Autodesk Inventor part; units mm, degrees
ref_plane "YZ Plane" through (0, 0, 0) normal (1, 0, 0) x (0, 1, 0)
ref_plane "XZ Plane" through (0, 0, 0) normal (0, 1, 0) x (-1, 0, 0)
ref_plane "XY Plane" through (0, 0, 0) normal (0, 0, 1) x (1, 0, 0)
sketch "Sketch1" plane through (0, 0, 0) normal (0, 1, 0) x (-1, 0, 0)
  line L0 (0, 0) -> (-30.48, 0)
  line L1 (-30.48, 0) -> (-30.48, -15.24)
  line L2 (-30.48, -15.24) -> (0, -15.24)
  line L3 (0, -15.24) -> (0, 0)
  line L4 (0, -7.62) -> (-30.48, -7.62) construction
  circle A0 centre (-7.874, -7.62) radius 1.143
  circle A1 centre (-22.606, -7.62) radius 1.143
  dimension "d0" = 15.24
  dimension "d1" = 30.48
  dimension "d2" = 2.286
  dimension "d3" = 2.286
  dimension "d4" = 14.732
  dimension "d5" = 7.874
extrude "Extrusion1" add sketch "Sketch1" along normal blind 2.032
sketch "Sketch2" plane through (0, 2.032, 0) normal (0, 1, 0) x (1, 0, 0)
  line L0 (0, 0) -> (30.48, 0)
  line L1 (30.48, 0) -> (30.48, 15.24)
  line L2 (30.48, 15.24) -> (0, 15.24)
  line L3 (0, 15.24) -> (0, 0)
  line L4 (2.032, 2.032) -> (28.448, 2.032)
  line L5 (28.448, 2.032) -> (28.448, 13.208)
  line L6 (28.448, 13.208) -> (2.032, 13.208)
  line L7 (2.032, 13.208) -> (2.032, 2.032)
  dimension "d8" = 2.032
  dimension "d9" = 2.032
  dimension "d10" = 2.032
  dimension "d12" = 2.032
extrude "Extrusion2" add sketch "Sketch2" along normal blind 0.9398
properties part number "castor_bracket"
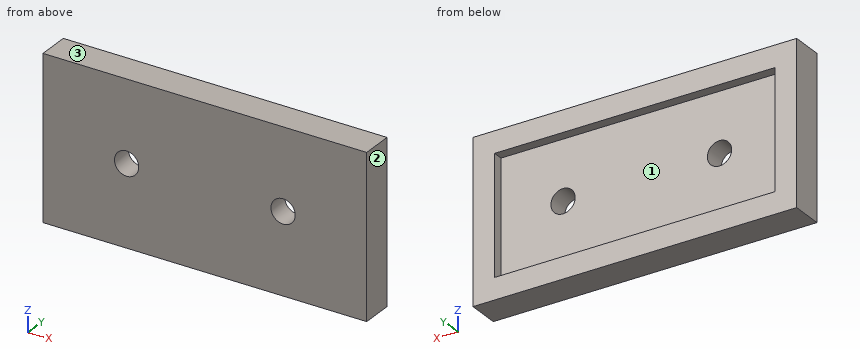
Design review of the part built by this model. Coordinates are the model's own, in mm. Face numbers are marked on the shaded views. Round coordinates to 2 decimals unless told otherwise and drop trailing zeros. Loops run counter-clockwise (first coordinate to the right, second up) from the corner with the lowest first, then second, coordinate; pieces in that order, holes last. Notation, with made-up numbers: (35, 19.5) -> (58, 19.5) arc R23 ccw to (58, 58.5) -> close; hole circle Ø11 at (77.25, -33.5). An arc over 180 degrees is marked (long way). Use one line per item in the form item = value. Start each with the question number.
Q1. We need section A-A on z = -7.62. Give the boundary of the cut face in (x, y).
Q2. We need section B-B on x = 22. Give the boundary of the cut face in (y, z).
Q3. We need section D-D on y = 2.35. Give the boundary of the cut face in (x, z).
Q4. Wall thickness on line 1 along Z through (x, y) = (23.5, 2.8); line 2 along Y through (x, z) = (11.5, -12.25): over which ranges is each line inside the solid? List them lowest first. Write a range as [from, to].
Q5. For pin 1 Ø3 at (x, z) = (6, -10) entering from +Y; pin 2 Ø8 at (x, z) = (25.5, -8) entering from -Y; pin 3 Ø1.4 at (x, z) = (22.606, -7.62) entering from -Y (3 decimals), all flat-tipped, find the tip position at first contact; note any pin that passes through.
Q6. We need section C-C on y = 1.05. Give the boundary of the cut face in (x, z).
Q7. Draft analysis for pull direction Z (two halves, no side actions). For the marked faces 1, 2 and 3, state which applies: +Z half, -Z half, draft (parallel to the pull), parting line (faces both ways), or undercut.
Calculated:
q1.outline = (0, 0) -> (6.73, 0) -> (6.73, 2.03) -> (2.03, 2.03) -> (2.03, 2.97) -> (0, 2.97) -> close; (9.02, 0) -> (21.46, 0) -> (21.46, 2.03) -> (9.02, 2.03) -> close; (23.75, 0) -> (30.48, 0) -> (30.48, 2.97) -> (28.45, 2.97) -> (28.45, 2.03) -> (23.75, 2.03) -> close
q2.outline = (0, -15.24) -> (2.97, -15.24) -> (2.97, -13.21) -> (2.03, -13.21) -> (2.03, -8.59) -> (0, -8.59) -> close; (0, -6.65) -> (2.03, -6.65) -> (2.03, -2.03) -> (2.97, -2.03) -> (2.97, 0) -> (0, 0) -> close
q3.outline = (0, -15.24) -> (30.48, -15.24) -> (30.48, 0) -> (0, 0) -> close; hole (2.03, -13.21) -> (28.45, -13.21) -> (28.45, -2.03) -> (2.03, -2.03) -> close
q4.line_1 = [-15.24, -13.21], [-2.03, 0]
q4.line_2 = [0, 2.03]
q5.pin_1 = 2.03
q5.pin_2 = 0
q5.pin_3 = through
q6.outline = (0, -15.24) -> (30.48, -15.24) -> (30.48, 0) -> (0, 0) -> close; hole circle Ø2.29 at (7.87, -7.62); hole circle Ø2.29 at (22.61, -7.62)
q7.face_1 = undercut
q7.face_2 = draft
q7.face_3 = +Z half
